Job drawing, mm, ordinate dimensions from the low corner. One solid piece. Give positions to 0.01 mm unless a question says otherwise; leave off trailing zeros. Write each loop counter-clockwise with the first axis right and the second up, starting at its lowest first coordinate (ties: lowest second). Pieces come first, ordered by that corner, then holes. Notation, with made-up numbers: (-9.5, 62) - (15.5, 62) arc R11 ccw to (15.5, 83) - close; hole circle Ø8 at (-39.75, 82). An arc over 180 degrees is marked (long way). Answer as a JSON object with one key per item and string values.
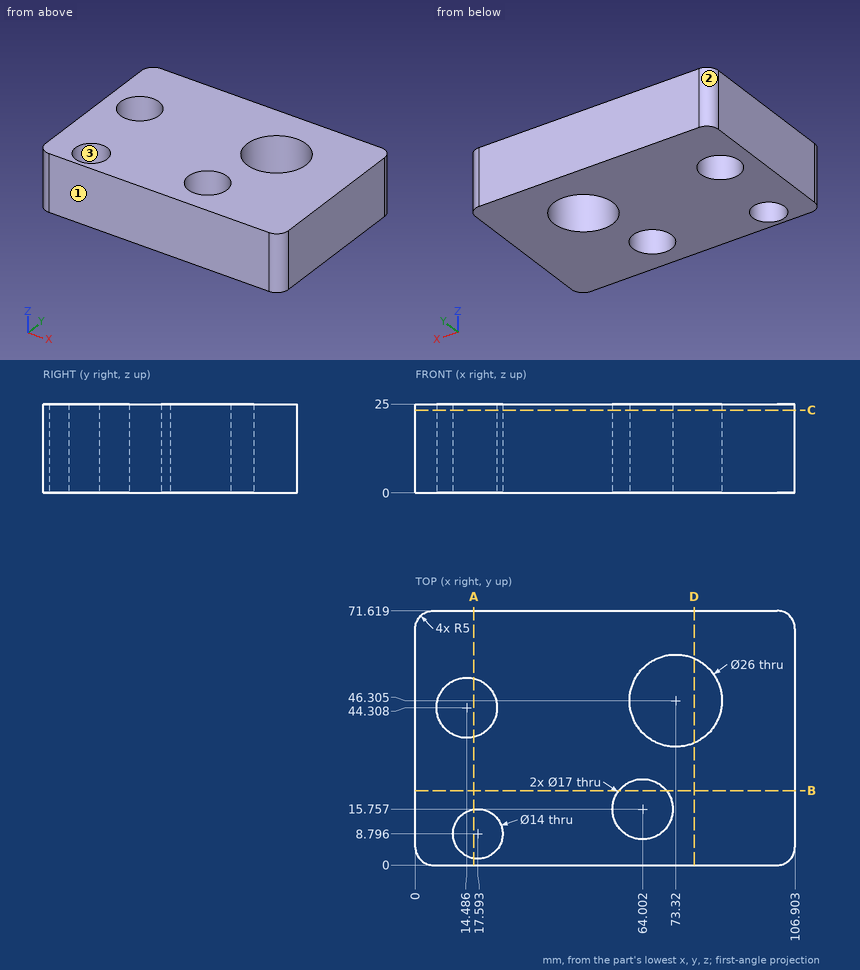
Item 1: Cut at B-B (y = 21). Give the cut face in (x, z).
Entries:
{"outline": "(0, 0) - (57.31, 0) - (57.31, 25) - (0, 25) - close; (70.69, 0) - (106.9, 0) - (106.9, 25) - (70.69, 25) - close"}
Item 2: Cut at C-C (z = 23.25). Give the cut face in (x, y) (1 decimal).
Entries:
{"outline": "(0, 5) arc R5 ccw to (5, 0) - (101.9, 0) arc R5 ccw to (106.9, 5) - (106.9, 66.6) arc R5 ccw to (101.9, 71.6) - (5, 71.6) arc R5 ccw to (0, 66.6) - close; hole circle Ø17 at (14.5, 44.3); hole circle Ø14 at (17.6, 8.8); hole circle Ø17 at (64, 15.8); hole circle Ø26 at (73.3, 46.3)"}
Item 3: Probe line 1 (X direction, y = 48.5, z = 12.75) (1 decimal); line 2 (Y direction, x = 68.5, z = 3.25) (1 decimal); line 3 (Y direction, x = 79.5, z = 3.25). List the from-to ranges inside material, lowest first. Write a range as from..to.
Entries:
{"line 1": "0..7.1, 21.9..60.5, 86.1..106.9", "line 2": "0..8.5, 23..34.2, 58.4..71.6", "line 3": "0..34.87, 57.74..71.62"}
Item 4: Mould opens along Y. For the marked faces 1, 2 and 3 say: +Y half, -Y half, draft (parallel to the pull), parting line (faces both ways), or undercut.
Entries:
{"face 1": "-Y half", "face 2": "+Y half", "face 3": "undercut"}
Item 5: Cut at D-D (x = 78.5). Give the cut face in (y, z).
Entries:
{"outline": "(0, 0) - (34.38, 0) - (34.38, 25) - (0, 25) - close; (58.23, 0) - (71.62, 0) - (71.62, 25) - (58.23, 25) - close"}
Item 6: Cut at A-A (x = 16.5). Give the cut face in (y, z).
Entries:
{"outline": "(0, 0) - (1.88, 0) - (1.88, 25) - (0, 25) - close; (15.71, 0) - (36.05, 0) - (36.05, 25) - (15.71, 25) - close; (52.57, 0) - (71.62, 0) - (71.62, 25) - (52.57, 25) - close"}
